Build history of the part. All positions in model axes, mm. A direction names the side the tool comes from. Round coordinates to 2 decimals unless told otherwise and drop trailing zeros. Order: outer loops, then holes, each group sorted by start corner. A loop starts at its lowest first (then second) coordinate and runs counter-clockwise, first axis right, second up. Notation, with made-up numbers: (58, -17) -> (104, -17) arc R27 ccw to (104, 3) -> close; hole circle Ø9 at (33, -23). An arc over 180 degrees is marked (long way). Write item = value, one per line.
from build123d import *

# Parameters (mm, degrees)
SKETCH_1_R          = 1
EXTRUDE_1_DEPTH     = 7
EXTRUDE_1_2_DEPTH   = 7
EXTRUDE_1_3_DEPTH   = 7
EXTRUDE_1_4_DEPTH   = 7
EXTRUDE_START       = -4
SKETCH_1_3_R        = 17.5
SKETCH_1_3_R_2      = 15
SKETCH_1_3_R_3      = 1
EXTRUDE_2_DEPTH     = 4
CUT_EXTRUDE_1_DEPTH = 3


with BuildPart() as part:
    # Sketch 1 → Extrude 1 (new body)
    with BuildSketch(Plane.XY):
        with BuildLine():
            Line((-10, 8.75), (-12.183492931, 8.75))
            ThreePointArc((-12.183492931, 8.75), (-15, 0), (-12.183492931, -8.75))
            Line((-12.183492931, -8.75), (-10, -8.75))
            Line((-10, -8.75), (-10, 8.75))
        make_face()
        with Locations((-12.5, 0)):
            Circle(SKETCH_1_R, mode=Mode.SUBTRACT)
    extrude(amount=EXTRUDE_1_DEPTH)



with BuildPart() as body_2:
    # Sketch 1 → Extrude 1 2 (new body)
    with BuildSketch(Plane.XY):
        with BuildLine():
            Line((-8.75, 12.183492931), (-8.75, 10))
            Line((-8.75, 10), (8.75, 10))
            Line((8.75, 10), (8.75, 12.183492931))
            ThreePointArc((8.75, 12.183492931), (0, 15), (-8.75, 12.183492931))
        make_face()
        with Locations((0, 12.5)):
            Circle(SKETCH_1_R, mode=Mode.SUBTRACT)
    extrude(amount=EXTRUDE_1_2_DEPTH)


with BuildPart() as body_3:
    # Sketch 1 → Extrude 1 3 (new body)
    with BuildSketch(Plane.XY):
        with BuildLine():
            ThreePointArc((15, 0), (14.278522227, 4.596063861), (12.183492931, 8.75))
            Line((12.183492931, 8.75), (10, 8.75))
            Line((10, 8.75), (10, -8.75))
            Line((10, -8.75), (12.183492931, -8.75))
            ThreePointArc((12.183492931, -8.75), (14.278522227, -4.596063861), (15, 0))
        make_face()
        with Locations((12.5, 0)):
            Circle(SKETCH_1_R, mode=Mode.SUBTRACT)
    extrude(amount=EXTRUDE_1_3_DEPTH)


with BuildPart() as body_4:
    # Sketch 1 → Extrude 1 4 (new body)
    with BuildSketch(Plane.XY):
        with BuildLine():
            Line((-8.75, -10), (-8.75, -12.183492931))
            ThreePointArc((-8.75, -12.183492931), (0, -15), (8.75, -12.183492931))
            Line((8.75, -12.183492931), (8.75, -10))
            Line((8.75, -10), (-8.75, -10))
        make_face()
        with Locations((0, -12.5)):
            Circle(SKETCH_1_R, mode=Mode.SUBTRACT)
    extrude(amount=EXTRUDE_1_4_DEPTH)


with BuildPart() as part_1:
    add(part.part)

    add(body_2.part)  # Extrude 2 merges body 2

    add(body_3.part)  # Extrude 2 merges body 3

    add(body_4.part)  # Extrude 2 merges body 4
    # Sketch 1_3 → Extrude 2 (add)
    # profile 1 of 5: a face of its own
    with BuildSketch(Plane.XY.offset(EXTRUDE_START)):
        Circle(SKETCH_1_3_R)
        Circle(SKETCH_1_3_R_2, mode=Mode.SUBTRACT)
    # profile 2 of 5: a face of its own
    with BuildSketch(Plane.XY.offset(EXTRUDE_START)):
        with BuildLine():
            Line((-8.75, 12.183492931), (-8.75, 10))
            Line((-8.75, 10), (8.75, 10))
            Line((8.75, 10), (8.75, 12.183492931))
            ThreePointArc((8.75, 12.183492931), (0, 15), (-8.75, 12.183492931))
        make_face()
        with Locations((0, 12.5)):
            Circle(SKETCH_1_3_R_3, mode=Mode.SUBTRACT)
    # profile 3 of 5: a face of its own
    with BuildSketch(Plane.XY.offset(EXTRUDE_START)):
        with BuildLine():
            ThreePointArc((15, 0), (14.278522227, 4.596063861), (12.183492931, 8.75))
            Line((12.183492931, 8.75), (10, 8.75))
            Line((10, 8.75), (10, -8.75))
            Line((10, -8.75), (12.183492931, -8.75))
            ThreePointArc((12.183492931, -8.75), (14.278522227, -4.596063861), (15, 0))
        make_face()
        with Locations((12.5, 0)):
            Circle(SKETCH_1_3_R_3, mode=Mode.SUBTRACT)
    # profile 4 of 5: a face of its own
    with BuildSketch(Plane.XY.offset(EXTRUDE_START)):
        with BuildLine():
            Line((-8.75, -10), (-8.75, -12.183492931))
            ThreePointArc((-8.75, -12.183492931), (0, -15), (8.75, -12.183492931))
            Line((8.75, -12.183492931), (8.75, -10))
            Line((8.75, -10), (-8.75, -10))
        make_face()
        with Locations((0, -12.5)):
            Circle(SKETCH_1_3_R_3, mode=Mode.SUBTRACT)
    # profile 5 of 5: a face of its own
    with BuildSketch(Plane.XY.offset(EXTRUDE_START)):
        with BuildLine():
            Line((-10, 8.75), (-12.183492931, 8.75))
            ThreePointArc((-12.183492931, 8.75), (-15, 0), (-12.183492931, -8.75))
            Line((-12.183492931, -8.75), (-10, -8.75))
            Line((-10, -8.75), (-10, 8.75))
        make_face()
        with Locations((-12.5, 0)):
            Circle(SKETCH_1_3_R_3, mode=Mode.SUBTRACT)
    extrude(amount=EXTRUDE_2_DEPTH)

    # Sketch 2 → Cut-Extrude 1 (cut)
    with BuildSketch(Plane(origin=(0, 0, -4), x_dir=(-1, 0, 0), z_dir=(0, 0, -1))):
        Polygon((10.5, -1.154700538), (12.5, -2.309401077), (14.5, -1.154700538), (14.5, 1.154700538), (12.5, 2.309401077), (10.5, 1.154700538), align=None)
        Polygon((1.154700538, 10.5), (2.309401077, 12.5), (1.154700538, 14.5), (-1.154700538, 14.5), (-2.309401077, 12.5), (-1.154700538, 10.5), align=None)
        Polygon((-1.154700538, -10.5), (-2.309401077, -12.5), (-1.154700538, -14.5), (1.154700538, -14.5), (2.309401077, -12.5), (1.154700538, -10.5), align=None)
        Polygon((-10.5, 1.154700538), (-12.5, 2.309401077), (-14.5, 1.154700538), (-14.5, -1.154700538), (-12.5, -2.309401077), (-10.5, -1.154700538), align=None)
    extrude(amount=-CUT_EXTRUDE_1_DEPTH, mode=Mode.SUBTRACT)


solid = part_1.part
Q1. Cut at A-A, the plane x = 0. List the corners of the cut face in (y, z).
Check values:
outline = (-17.5, -4) -> (-14.5, -4) -> (-14.5, -1) -> (-13.5, -1) -> (-13.5, 7) -> (-15, 7) -> (-15, 0) -> (-17.5, 0) -> close; (-11.5, -1) -> (-10.5, -1) -> (-10.5, -4) -> (-10, -4) -> (-10, 7) -> (-11.5, 7) -> close; (10, -4) -> (10.5, -4) -> (10.5, -1) -> (11.5, -1) -> (11.5, 7) -> (10, 7) -> close; (13.5, -1) -> (14.5, -1) -> (14.5, -4) -> (17.5, -4) -> (17.5, 0) -> (15, 0) -> (15, 7) -> (13.5, 7) -> close
Q2. Cut at D-D, the plane x = -4.5. List the corners of the cut face in (y, z), and give its area (3 significant figures).
Check values:
outline = (-16.91, -4) -> (-10, -4) -> (-10, 7) -> (-14.31, 7) -> (-14.31, 0) -> (-16.91, 0) -> close; (10, -4) -> (16.91, -4) -> (16.91, 0) -> (14.31, 0) -> (14.31, 7) -> (10, 7) -> close
area = 116 mm²
Q3. Cut at B-B, the plane z = 0.75. List the corners of the cut face in (x, y).
Check values:
outline = (-12.18, -8.75) -> (-10, -8.75) -> (-10, 8.75) -> (-12.18, 8.75) arc R15 ccw to start; (-8.75, -12.18) arc R15 ccw to (8.75, -12.18) -> (8.75, -10) -> (-8.75, -10) -> close; (-8.75, 10) -> (8.75, 10) -> (8.75, 12.18) arc R15 ccw to (-8.75, 12.18) -> close; (10, -8.75) -> (12.18, -8.75) arc R15 ccw to (12.18, 8.75) -> (10, 8.75) -> close; hole circle Ø2 at (-12.5, 0); hole circle Ø2 at (0, -12.5); hole circle Ø2 at (0, 12.5); hole circle Ø2 at (12.5, 0)
Q4. Flat gauge pins, fed straight in: pin 1 (1.1 mm diameter, centred on y = 11.5, z = -0.5, fed in from -X); pin 2 (1.6 mm diameter, centred on x = 12.5, y = 0, fed in from -Z); pin 3 (5 mm diameter, centred on x = 8.5, z = -0.5, fed in from -Y); pin 4 (3.5 mm diameter, centred on x = 4, z = 1, fed in from +Y). Where does each tip first touch, or does it go through?
Check values:
pin_1 = -13.65
pin_2 = through
pin_3 = -16.44
pin_4 = 17.31
Q5. Cut at C-C, the plane y = -8. List the corners of the cut face in (x, z), and give its area (3 significant figures).
Check values:
outline = (-15.56, -4) -> (-10, -4) -> (-10, 7) -> (-12.69, 7) -> (-12.69, 0) -> (-15.56, 0) -> close; (10, -4) -> (15.56, -4) -> (15.56, 0) -> (12.69, 0) -> (12.69, 7) -> (10, 7) -> close
area = 82.2 mm²
Q6. Probe probe 1 along Y at (x, z) = (12.5, 0.5); probe 2 along Y at (x, z) = (1.5, 3.75); probe 3 along X at (y, z) = (13, 2.75). List the from-to ranges inside material, lowest first.
Check values:
probe_1 = -8.29 to -1, 1 to 8.29
probe_2 = -14.92 to -10, 10 to 14.92
probe_3 = -7.48 to -0.87, 0.87 to 7.48
Q7. Mould opens along X. For faces 4 (the face through (11, 0, 7)), 5 (the face through (0, 14.5, -3)) say: released by +X, released by -X, zero draft, split by the parting line, or undercut.
Check values:
face_4 = zero draft
face_5 = undercut
Q8. Which spindle directions (+Z, -Z, +X, -X, +Y, -Y) get a long thin tool onto all of the face, cutting with end or side? Do faces 1 (the face through (13, 8, 0)), 2 (the face through (0, 10, 1)), 3 (the face through (1.724, -11.486, -2.521)). Say none if no direction does.
Check values:
face_1 = +Z
face_2 = +Z, -Z
face_3 = -Z
